The model under review builds one solid part; all positions refer to its coordinate system, in mm. Give positions to 0.01 mm unless a question says otherwise; leave off trailing zeros. Loops run counter-clockwise (first coordinate to the right, second up) from the corner with the lowest first, then second, coordinate; pieces in that order, holes last. Notation, with made-up numbers: M 53,43 L 101,43 A15 cw 101,63 Z; hole C 62.25,78.5 d6. An arc over 180 degrees is marked long. Write item = value, one per line. Start each with the question number.
1. We need section A-A on x = 0. Give the boundary of the cut face in (y, z), then the cut area to 3 significant figures.
2. For pin 1 (2 mm diameter, centred on y = 18.5, z = -44.5, fed in from -X); pin 2 (12 mm diameter, centred on y = -58.5, z = -35.5, fed in from -X); pin 3 (3 mm diameter, centred on x = -68, y = -73.5, fed in from -Z); pin 4 (1.7 mm diameter, centred on x = -28, y = 97.5, fed in from -Z), all flat-tipped, find the tip position at first contact; note any pin that passes through.
3. Wall thickness on line 1 along Y through (x, z) = (1.5, -90); line 2 along X through (y, z) = (13, -73); line 3 along Y through (x, z) = (4.5, -74): over which ranges is each line inside the solid? List them lowest first. Write a range as from..to.
4. Draft analysis for pull direction Y (two halves, no side actions). For faces 1 (the face through (-8.67, -39.05, -49.37)), 2 (the face through (1, 47, 0)), state which applies: pulls with the +Y half, pulls with the -Y half, needs draft (parallel to the pull), parting line crosses it, or undercut.
from build123d import *

# Parameters (mm, degrees)
SKETCH2_R           = 100
SKETCH2_R_2         = 50
BOSS_EXTRUDE2_DEPTH = 100
SKETCH3_R           = 50
BOSS_EXTRUDE3_DEPTH = 100
SKETCH4_R           = 40
CUT_EXTRUDE1_DEPTH  = 100
FILLET1_R           = 5
FILLET2_R           = 5
BOSS_EXTRUDE4_DEPTH = 99


with BuildPart() as part:
    # Sketch2 → Boss-Extrude2 (new body)
    with BuildSketch(Plane.XY):
        Circle(SKETCH2_R)
        Circle(SKETCH2_R_2, mode=Mode.SUBTRACT)
    extrude(amount=-BOSS_EXTRUDE2_DEPTH)

    # Sketch3 → Boss-Extrude3 (add)
    with BuildSketch(Plane.XY):
        Circle(SKETCH3_R)
    extrude(amount=-BOSS_EXTRUDE3_DEPTH)

    # Sketch4 → Cut-Extrude1 (cut)
    with BuildSketch(Plane.XY):
        Circle(SKETCH4_R)
    extrude(amount=-CUT_EXTRUDE1_DEPTH, mode=Mode.SUBTRACT)

    # Fillet1
    fillet1_edges = [part.edges().sort_by_distance(p)[0] for p in [
        (-40, 0, 0),
    ]]
    fillet(fillet1_edges, radius=FILLET1_R)

    # Fillet2
    fillet2_edges = [part.edges().sort_by_distance(p)[0] for p in [
        (-40, 0, -100),
    ]]
    fillet(fillet2_edges, radius=FILLET2_R)

    # Sketch9 → Boss-Extrude4 (add)
    with BuildSketch(Plane.XY):
        with BuildLine():
            Line((-11.094188182, 99.382689582), (-8.236971303, 102.239906461))
            Line((-8.236971303, 102.239906461), (-5.827142523, 99.830077682))
            ThreePointArc((-5.827142523, 99.830077682), (-8.463621993, 99.641191797), (-11.094188182, 99.382689582))
        make_face()
        with BuildLine():
            Line((13.199898104, 101.718281835), (15.056034767, 98.86008202))
            ThreePointArc((15.056034767, 98.86008202), (12.437897116, 99.22347865), (9.811069477, 99.517550792))
            Line((9.811069477, 99.517550792), (13.199898104, 101.718281835))
        make_face()
        with BuildLine():
            Line((34.059868624, 96.751080194), (35.281191091, 93.569426391))
            ThreePointArc((35.281191091, 93.569426391), (32.795820437, 94.469223358), (30.287536321, 95.303017495))
            Line((30.287536321, 95.303017495), (34.059868624, 96.751080194))
        make_face()
        with BuildLine():
            Line((53.431259448, 87.555392086), (53.964390067, 84.189337833))
            ThreePointArc((53.964390067, 84.189337833), (51.720409033, 85.586209692), (49.440292492, 86.923285018))
            Line((49.440292492, 86.923285018), (53.431259448, 87.555392086))
        make_face()
        with BuildLine():
            Line((70.467447842, 74.533113206), (70.289086246, 71.129771226))
            ThreePointArc((70.289086246, 71.129771226), (68.384567572, 72.962667974), (66.43227064, 74.744587882))
            Line((66.43227064, 74.744587882), (70.467447842, 74.533113206))
        make_face()
        with BuildLine():
            Line((84.423870625, 58.253379629), (83.541812073, 54.961492298))
            ThreePointArc((83.541812073, 54.961492298), (82.059992363, 57.150307552), (80.520839784, 59.299193591))
            Line((80.520839784, 59.299193591), (84.423870625, 58.253379629))
        make_face()
        with BuildLine():
            Line((94.690565151, 39.427693832), (93.143359833, 36.391132422))
            ThreePointArc((93.143359833, 36.391132422), (92.14900172, 38.840204453), (91.090261847, 41.262139991))
            Line((91.090261847, 41.262139991), (94.690565151, 39.427693832))
        make_face()
        with BuildLine():
            Line((100.818827604, 18.878828619), (98.674095818, 16.230305435))
            ThreePointArc((98.674095818, 16.230305435), (98.210657522, 18.832598043), (97.678602368, 21.421732876))
            Line((97.678602368, 21.421732876), (100.818827604, 18.878828619))
        make_face()
        with BuildLine():
            Line((102.540823508, -2.495131995), (99.892300324, -4.639863781))
            ThreePointArc((99.892300324, -4.639863781), (99.980036323, -1.998083271), (99.997919252, 0.645093241))
            Line((99.997919252, 0.645093241), (102.540823508, -2.495131995))
        make_face()
        with BuildLine():
            Line((99.78129338, -23.760043368), (96.74473197, -25.307248685))
            ThreePointArc((96.74473197, -25.307248685), (97.37980778, -22.741438757), (97.946847221, -20.159740064))
            Line((97.946847221, -20.159740064), (99.78129338, -23.760043368))
        make_face()
        with BuildLine():
            Line((92.660841927, -43.986526832), (89.368954596, -44.868585384))
            ThreePointArc((89.368954596, -44.868585384), (90.523614356, -42.490884245), (91.615027965, -40.083495991))
            Line((91.615027965, -40.083495991), (92.660841927, -43.986526832))
        make_face()
        with BuildLine():
            Line((81.490667046, -62.290588003), (78.087325067, -62.468949599))
            ThreePointArc((78.087325067, -62.468949599), (79.711104604, -60.383274197), (81.27919237, -58.255410802))
            Line((81.27919237, -58.255410802), (81.490667046, -62.290588003))
        make_face()
        with BuildLine():
            Line((66.75895898, -77.872251575), (63.392904727, -77.339120956))
            ThreePointArc((63.392904727, -77.339120956), (65.414837085, -75.636625315), (67.391066047, -73.881284619))
            Line((67.391066047, -73.881284619), (66.75895898, -77.872251575))
        make_face()
        with BuildLine():
            Line((49.109564061, -90.050524081), (45.927910258, -88.829201614))
            ThreePointArc((45.927910258, -88.829201614), (48.25962729, -87.584292963), (50.55762676, -86.278191777))
            Line((50.55762676, -86.278191777), (49.109564061, -90.050524081))
        make_face()
        with BuildLine():
            Line((29.313845538, -98.293156574), (26.455645724, -96.437019911))
            ThreePointArc((26.455645724, -96.437019911), (28.995240207, -95.704106732), (31.514576581, -94.904327946))
            Line((31.514576581, -94.904327946), (29.313845538, -98.293156574))
        make_face()
        with BuildLine():
            Line((8.236971303, -102.239906461), (5.827142523, -99.830077682))
            ThreePointArc((5.827142523, -99.830077682), (8.463621993, -99.641191797), (11.094188182, -99.382689582))
            Line((11.094188182, -99.382689582), (8.236971303, -102.239906461))
        make_face()
        with BuildLine():
            Line((-13.199898104, -101.718281835), (-15.056034767, -98.86008202))
            ThreePointArc((-15.056034767, -98.86008202), (-12.437897116, -99.22347865), (-9.811069477, -99.517550792))
            Line((-9.811069477, -99.517550792), (-13.199898104, -101.718281835))
        make_face()
        with BuildLine():
            Line((-34.059868624, -96.751080194), (-35.281191091, -93.569426391))
            ThreePointArc((-35.281191091, -93.569426391), (-32.795820437, -94.469223358), (-30.287536321, -95.303017495))
            Line((-30.287536321, -95.303017495), (-34.059868624, -96.751080194))
        make_face()
        with BuildLine():
            Line((-53.431259448, -87.555392086), (-53.964390067, -84.189337833))
            ThreePointArc((-53.964390067, -84.189337833), (-51.720409033, -85.586209692), (-49.440292492, -86.923285018))
            Line((-49.440292492, -86.923285018), (-53.431259448, -87.555392086))
        make_face()
        with BuildLine():
            Line((-70.467447842, -74.533113206), (-70.289086246, -71.129771226))
            ThreePointArc((-70.289086246, -71.129771226), (-68.384567572, -72.962667974), (-66.43227064, -74.744587882))
            Line((-66.43227064, -74.744587882), (-70.467447842, -74.533113206))
        make_face()
        with BuildLine():
            Line((-84.423870625, -58.253379629), (-83.541812073, -54.961492298))
            ThreePointArc((-83.541812073, -54.961492298), (-82.059992363, -57.150307552), (-80.520839784, -59.299193591))
            Line((-80.520839784, -59.299193591), (-84.423870625, -58.253379629))
        make_face()
        with BuildLine():
            Line((-94.690565151, -39.427693832), (-93.143359833, -36.391132422))
            ThreePointArc((-93.143359833, -36.391132422), (-92.14900172, -38.840204453), (-91.090261847, -41.262139991))
            Line((-91.090261847, -41.262139991), (-94.690565151, -39.427693832))
        make_face()
        with BuildLine():
            Line((-100.818827604, -18.878828619), (-98.674095818, -16.230305435))
            ThreePointArc((-98.674095818, -16.230305435), (-98.210657522, -18.832598043), (-97.678602368, -21.421732875))
            Line((-97.678602368, -21.421732875), (-100.818827604, -18.878828619))
        make_face()
        with BuildLine():
            Line((-102.540823508, 2.495131995), (-99.892300324, 4.639863781))
            ThreePointArc((-99.892300324, 4.639863781), (-99.980036323, 1.998083271), (-99.997919252, -0.645093241))
            Line((-99.997919252, -0.645093241), (-102.540823508, 2.495131995))
        make_face()
        with BuildLine():
            Line((-99.78129338, 23.760043368), (-96.74473197, 25.307248685))
            ThreePointArc((-96.74473197, 25.307248685), (-97.37980778, 22.741438757), (-97.946847221, 20.159740064))
            Line((-97.946847221, 20.159740064), (-99.78129338, 23.760043368))
        make_face()
        with BuildLine():
            Line((-92.660841927, 43.986526832), (-89.368954596, 44.868585384))
            ThreePointArc((-89.368954596, 44.868585384), (-90.523614356, 42.490884245), (-91.615027965, 40.083495991))
            Line((-91.615027965, 40.083495991), (-92.660841927, 43.986526832))
        make_face()
        with BuildLine():
            Line((-81.490667046, 62.290588003), (-78.087325067, 62.468949599))
            ThreePointArc((-78.087325067, 62.468949599), (-79.711104604, 60.383274197), (-81.27919237, 58.255410802))
            Line((-81.27919237, 58.255410802), (-81.490667046, 62.290588003))
        make_face()
        with BuildLine():
            Line((-66.75895898, 77.872251575), (-63.392904727, 77.339120956))
            ThreePointArc((-63.392904727, 77.339120956), (-65.414837085, 75.636625315), (-67.391066047, 73.881284619))
            Line((-67.391066047, 73.881284619), (-66.75895898, 77.872251575))
        make_face()
        with BuildLine():
            Line((-49.109564061, 90.050524081), (-45.927910258, 88.829201614))
            ThreePointArc((-45.927910258, 88.829201614), (-48.25962729, 87.584292963), (-50.55762676, 86.278191777))
            Line((-50.55762676, 86.278191777), (-49.109564061, 90.050524081))
        make_face()
        with BuildLine():
            Line((-29.313845538, 98.293156574), (-26.455645724, 96.437019911))
            ThreePointArc((-26.455645724, 96.437019911), (-28.995240207, 95.704106732), (-31.514576581, 94.904327946))
            Line((-31.514576581, 94.904327946), (-29.313845538, 98.293156574))
        make_face()
    extrude(amount=-BOSS_EXTRUDE4_DEPTH)


solid = part.part
Final values:
q1.outline = M -100,-100 L -45,-100 A5 ccw -40,-95 L -40,-5 A5 ccw -45,0 L -100,0 Z; M 40,-95 A5 ccw 45,-100 L 100,-100 L 100,0 L 45,0 A5 ccw 40,-5 Z
q1.area = 12,000 mm²
q2.pin_1 = -98.46
q2.pin_2 = -85.11
q2.pin_3 = -100
q2.pin_4 = -99
q3.line_1 = -99.99..-39.97, 39.97..99.99
q3.line_2 = -99.15..-37.83, 37.83..99.15
q3.line_3 = -99.9..-39.75, 39.75..99.9
q4.face_1 = undercut
q4.face_2 = needs draft
